Check sheet for the modelled part. Datum: model origin and axes. Units: mm. Round coordinates to 2 decimals unless told otherwise and drop trailing zeros. Order: outer loops, then holes, each group sorted by start corner. A loop starts at its lowest first (then second) coordinate and runs counter-clockwise, first axis right, second up. Notation, with made-up numbers: (19, 23) -> (54, 23) arc R29 cw to (54, 49) -> close; hole circle Ø2 at (-4.5, -12.75). An arc over 180 degrees is marked (long way). Answer in a Markdown table with one row per item.
from build123d import *

# Parameters (mm, degrees)
SKETCH2_W           = 6
SKETCH2_H           = 240
BOSS_EXTRUDE1_DEPTH = 3
BOSS_EXTRUDE2_DEPTH = 240
SKETCH5_W           = 3
SKETCH5_H           = 3
BOSS_EXTRUDE3_DEPTH = 10


with BuildPart() as part:
    # Sketch2 → Boss-Extrude1 (new body)
    with BuildSketch(Plane.XY):
        with Locations((-3, -120)):
            Rectangle(SKETCH2_W, SKETCH2_H)
    extrude(amount=BOSS_EXTRUDE1_DEPTH)

    # Sketch4 → Boss-Extrude2 (add)
    with BuildSketch(Plane(origin=(0, -240, 0), x_dir=(-1, 0, 0), z_dir=(0, -1, 0))):
        Polygon((0, 0), (-2.828427125, 2.828427125), (-2.828427125, -3), (0, -3), align=None)
        Polygon((8.828427125, -3), (6, -3), (6, 0), (8.828427125, 2.828427125), align=None)
    extrude(amount=-BOSS_EXTRUDE2_DEPTH)

    # Sketch5 → Boss-Extrude3 (add)
    with BuildSketch(Plane(origin=(0, 0, 0), x_dir=(1, 0, 0), z_dir=(0, 1, 0))):
        with Locations((-6.5, -1.5)):
            Rectangle(SKETCH5_W, SKETCH5_H)
        with Locations((0.5, -1.5)):
            Rectangle(SKETCH5_W, SKETCH5_H)
    extrude(amount=BOSS_EXTRUDE3_DEPTH)


solid = part.part
Item 1: Cross-section at B-B (y = -208.5). Record the boundary of the cut face in (x, z).
Result sheet:
| item | result |
|---|---|
| outline | (-8.83, -2.83) -> (-6, 0) -> (0, 0) -> (2.83, -2.83) -> (2.83, 3) -> (-8.83, 3) -> close |
Item 2: Depth check by flat-ended pin: P1, Ø1.4, axis at x = -7, z = -1, coming from the +Y side; P2, Ø0.9, axis at y = 4, z = 1, coming from the -X side; P3, Ø5, axis at x = -4.5, y = -83.5, coming from the -Z side. Enter the tip coordinate at first touch or a pass-through.
Result sheet:
| item | result |
|---|---|
| P1 | stops at y = 0 |
| P2 | stops at x = -8 |
| P3 | stops at z = -1 |
Item 3: Scan lines: line 1 (Z direction, x = -3.25, y = -172); line 2 (X direction, y = -216, z = -2); line 3 (Y direction, x = 2.25, z = 0). Record each from-to range of solid material in increasing order. Write a range as [from, to].
Result sheet:
| item | result |
|---|---|
| line 1 | z = [0, 3] |
| line 2 | x = [-8.83, -8], [2, 2.83] |
| line 3 | y = [-240, 0] |
Item 4: Mould release check, pull along X, two halves, no side actions. Record for faces 1 (the flat face through (2.828, -122, 0)), 2 (the flat face through (-3, -240, 1)), 3 (the flat face through (-3, -117, 0)): pulls with the +X half, pulls with the -X half, needs draft (parallel to the pull), parting line crosses it, or undercut.
Result sheet:
| item | result |
|---|---|
| face 1 | pulls with the +X half |
| face 2 | needs draft |
| face 3 | undercut |
Item 5: Cross-section at A-A (z = -1). Record the boundary of the cut face in (x, y).
Result sheet:
| item | result |
|---|---|
| outline | (-8.83, -240) -> (-7, -240) -> (-7, 0) -> (-8.83, 0) -> close; (1, -240) -> (2.83, -240) -> (2.83, 0) -> (1, 0) -> close |
